Design review of the part built by this model. Coordinates are the model's own, in mm. Face numbers are marked on the shaded views. Coordinates: 2 decimals unless noted, no trailing zeros. Write each loop counter-clockwise with the first axis right and the second up, starting at its lowest first coordinate (ties: lowest second). Pieces come first, ordered by that corner, then holes. Notation, with made-up numbers: (35.5, 41) - (56.5, 41) arc R20 cw to (56.5, 67) - close; hole circle Ø11 at (2, -37). An arc over 180 degrees is marked (long way). One line per item, written item: value.
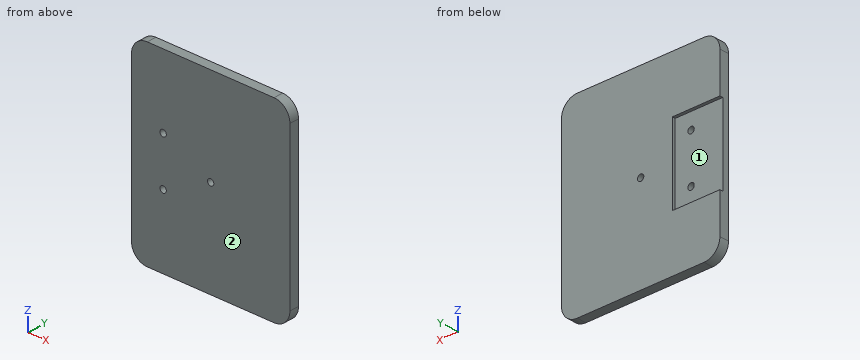
from build123d import *

# Parameters (mm, degrees)
SKETCH1_R           = 1
BOSS_EXTRUDE1_DEPTH = 3
SKETCH2_W           = 15
SKETCH2_H           = 25
CUT_EXTRUDE1_DEPTH  = 1


with BuildPart() as part:
    # Sketch1 → Boss-Extrude1 (new body)
    with BuildSketch(Plane(origin=(0, 0, 0), x_dir=(1, 0, 0), z_dir=(0, 1, 0))):
        with BuildLine():
            Line((-52.254901961, 26.274509804), (-12.254901961, 26.274509804))
            ThreePointArc((-12.254901961, 26.274509804), (-8.719368055, 24.81004371), (-7.254901961, 21.274509804))
            Line((-7.254901961, 21.274509804), (-7.254901961, -28.725490196))
            ThreePointArc((-7.254901961, -28.725490196), (-8.719368055, -32.261024102), (-12.254901961, -33.725490196))
            Line((-12.254901961, -33.725490196), (-52.254901961, -33.725490196))
            ThreePointArc((-52.254901961, -33.725490196), (-55.790435867, -32.261024102), (-57.254901961, -28.725490196))
            Line((-57.254901961, -28.725490196), (-57.254901961, 21.274509804))
            ThreePointArc((-57.254901961, 21.274509804), (-55.790435867, 24.81004371), (-52.254901961, 26.274509804))
        make_face()
        with Locations(Location((-32.254901961, -3.725490196, 0), (0, 0, 270))):
            Circle(SKETCH1_R, mode=Mode.SUBTRACT)
        with Locations(Location((-47.254901961, 3.774509804, 0), (0, 0, 270))):
            Circle(SKETCH1_R, mode=Mode.SUBTRACT)
        with Locations(Location((-47.254901961, -11.225490196, 0), (0, 0, 270))):
            Circle(SKETCH1_R, mode=Mode.SUBTRACT)
    extrude(amount=BOSS_EXTRUDE1_DEPTH)

    # Sketch2 → Cut-Extrude1 (cut)
    with BuildSketch(Plane(origin=(0, 3, 0), x_dir=(1, 0, 0), z_dir=(0, 1, 0))):
        with Locations((-49.754901961, -3.725490196)):
            Rectangle(SKETCH2_W, SKETCH2_H)
    extrude(amount=-CUT_EXTRUDE1_DEPTH, mode=Mode.SUBTRACT)


solid = part.part
1. Insertion check: pin 1 Ø0.5 at (y, z) = (2.5, -1) entering from -X; pin 2 Ø1.8 at (x, z) = (-47.25, 11.23) entering from +Y; pin 3 Ø7.5 at (x, z) = (-46.5, 0.5) entering from +Y. Each pin has a flat end and moves straight along its axis. Give the tip position at first contact, or say it passes through.
Answer block:
pin 1: stops at x = -42.25
pin 2: passes through
pin 3: stops at y = 2
2. Wall thickness on line 1 along X through (y, z) = (2.5, 4.5); line 2 along Z through (x, y) = (-31.5, 1.3); line 3 along X through (y, z) = (2.1, 4): over which ranges is each line inside the solid? List them lowest first.
Answer block:
line 1: x = -42.25 to -32.89, -31.62 to -7.25
line 2: z = -26.27 to 3.07, 4.38 to 33.73
line 3: x = -42.25 to -33.22, -31.29 to -7.25
3. Mouldability with a two-part tool opening along Z and no side actions: class the marked faces 1 and 2 as released by +Z, released by -Z, zero draft, split by the parting line, or undercut.
Answer block:
face 1: undercut
face 2: zero draft
4. Consider section A-A, the plane z = 3.5. Write out the cut boundary in (x, y), then the cut area to 3 significant figures.
Answer block:
outline: (-57.25, 0) - (-33.23, 0) - (-33.23, 3) - (-42.25, 3) - (-42.25, 2) - (-57.25, 2) - close; (-31.28, 0) - (-7.25, 0) - (-7.25, 3) - (-31.28, 3) - close
area: 129 mm^2
